Read the model definition and answer for the solid it produces. Units are mm, in the model's axes. Give positions to 0.01 mm unless a question says otherwise; leave off trailing zeros. Loops run counter-clockwise (first coordinate to the right, second up) from the corner with the lowest first, then second, coordinate; pieces in that order, holes last. Notation, with made-up numbers: (-37, -19) - (-23, -19) arc R23 cw to (-23, -9) - close; hole circle Ø11 at (2, 45). An arc over 180 degrees is marked (long way). Use a Markdown table: item, result. Add a question column.
Item 1: A cutting plane is placed at B-B (z = 26). Determine the outline of the cut face in (x, y), plus the area to 3 significant figures.
Item 2: A cutting plane is placed at A-A (x = 37). Determine the outline of the cut face in (y, z).
Item 3: A cutting plane is placed at C-C (y = 1.2). Determine the outline of the cut face in (x, z), plus the area to 3 significant figures.
Item 4: Consider probe 1 along X at (y, z) = (1.5, 28.4); probe 2 along Z at (x, y) = (43.15, 1.1); probe 3 along Z at (x, y) = (31, 0.3). Determine where each line is inside the solid, lowest interval first. Write a range as [from, to].
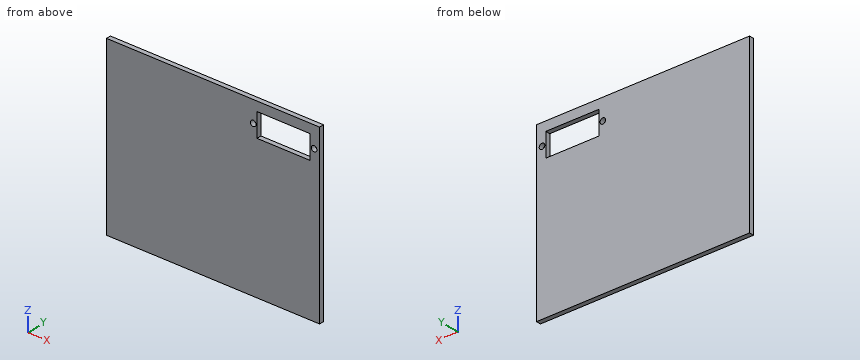
from build123d import *

# Parameters (mm, degrees)
SKETCH_1_W          = 91
SKETCH_1_H          = 75
EXTRUDE_1_DEPTH     = 2
SKETCH_2_R          = 1.2
SKETCH_2_W          = 22.7
SKETCH_2_H          = 10.2
CUT_EXTRUDE_1_DEPTH = 2


with BuildPart() as part:
    # 草图1 → 凸台-拉伸1 (new body)
    with BuildSketch(Plane(origin=(0, 0, 0), x_dir=(1, 0, 0), z_dir=(0, 1, 0))):
        Rectangle(SKETCH_1_W, SKETCH_1_H)
    extrude(amount=EXTRUDE_1_DEPTH)

    # 草图2 → 切除-拉伸1 (cut)
    with BuildSketch(Plane(origin=(0, 2, 0), x_dir=(1, 0, 0), z_dir=(0, 1, 0))):
        with Locations(Location((17.15, -28.4, 0), (0, 0, 270))):
            Circle(SKETCH_2_R)
        with Locations(Location((43.15, -28.4, 0), (0, 0, 90))):
            Circle(SKETCH_2_R)
        with Locations((30.15, -28.4)):
            Rectangle(SKETCH_2_W, SKETCH_2_H)
    extrude(amount=-CUT_EXTRUDE_1_DEPTH, mode=Mode.SUBTRACT)


solid = part.part
Geometry says:
| question | item | result |
|---|---|---|
| 1 | outline | (-45.5, 0) - (18.8, 0) - (18.8, 2) - (-45.5, 2) - close; (41.5, 0) - (45.5, 0) - (45.5, 2) - (41.5, 2) - close |
| 1 | area | 137 mm² |
| 2 | outline | (0, -37.5) - (2, -37.5) - (2, 23.3) - (0, 23.3) - close; (0, 33.5) - (2, 33.5) - (2, 37.5) - (0, 37.5) - close |
| 3 | outline | (-45.5, -37.5) - (45.5, -37.5) - (45.5, 37.5) - (-45.5, 37.5) - close; hole circle Ø2.4 at (17.15, 28.4); hole (18.8, 23.3) - (41.5, 23.3) - (41.5, 33.5) - (18.8, 33.5) - close; hole circle Ø2.4 at (43.15, 28.4) |
| 3 | area | 6,580 mm² |
| 4 | probe 1 | [-45.5, 15.95], [18.35, 18.8], [41.5, 41.95], [44.35, 45.5] |
| 4 | probe 2 | [-37.5, 27.2], [29.6, 37.5] |
| 4 | probe 3 | [-37.5, 23.3], [33.5, 37.5] |
